Geometry: final body of the model. Coordinates: model frame, mm. Give positions to 0.01 mm unless a question says otherwise; leave off trailing zeros. Order: outer loops, then holes, each group sorted by start corner. A loop starts at its lowest first (then second) coordinate and runs counter-clockwise, first axis right, second up. Notation, with made-up numbers: M 75.25,74.25 L 106.25,74.25 A26 cw 106.25,96.25 Z; hole C 88,-24.5 d11. An arc over 180 degrees is marked long. Use CSV: the item, a comma, the result in double quotes.
Autodesk Inventor part; units mm, degrees
ref_plane "YZ Plane" through (0, 0, 0) normal (1, 0, 0) x (0, 1, 0)
ref_plane "XZ Plane" through (0, 0, 0) normal (0, 1, 0) x (-1, 0, 0)
ref_plane "XY Plane" through (0, 0, 0) normal (0, 0, 1) x (1, 0, 0)
sketch "スケッチ1" plane through (0, 0, 0) normal (0, 1, 0) x (-1, 0, 0)
  line L0 (127.92, 0) -> (-21.32, 0)
  line L1 (0, -84) -> (0, 84)
  line L2 (106.6, 0) -> (106.6, -60)
  line L3 (106.6, -60) -> (0, -60)
  line L4 (0, -40) -> (86.6, -40)
  line L5 (86.6, -40) -> (86.6, 0)
  line L6 (106.6, 0) -> (106.6, 60)
  line L7 (106.6, 60) -> (0, 60)
  line L8 (0, 40) -> (86.6, 40)
  line L9 (86.6, 40) -> (86.6, 0)
  line L10 (0, 60) -> (0, 40)
  line L11 (0, -40) -> (0, -60)
  point P0 (0, 0)
  dimension "d0" = 20
  dimension "d4" = 20
  dimension "d15" = 60
  dimension "d16" = 106.6
extrude "押し出し1" add sketch "スケッチ1" along normal blind 5 contours L2 L3 L1 L4 L5 L0 | L0 L9 L8 L1 L7 L6
sketch "スケッチ2" plane through (0, 5, 0) normal (0, 1, 0) x (1, 0, 0)
  circle A0 centre (-10, -50) radius 5
  line L0 (0, -60) -> (0, -40)
  line L1 (-106.6, -60) -> (0, -60)
  line L2 (-127.92, 0) -> (21.32, 0)
  circle A1 centre (-10, 50) radius 5
  circle A2 centre (-96.6, 0) radius 5
  line L3 (-86.6, -40) -> (-86.6, 40)
  point P0 (0, 0)
  dimension "d8" = 10
  dimension "d9" = 10
  dimension "d10" = 10
  dimension "d11" = 10
  dimension "d12" = 10
extrude "押し出し2" cut sketch "スケッチ2" against normal blind 5
properties part number "bogie_square" material "アルミニウム 6061"
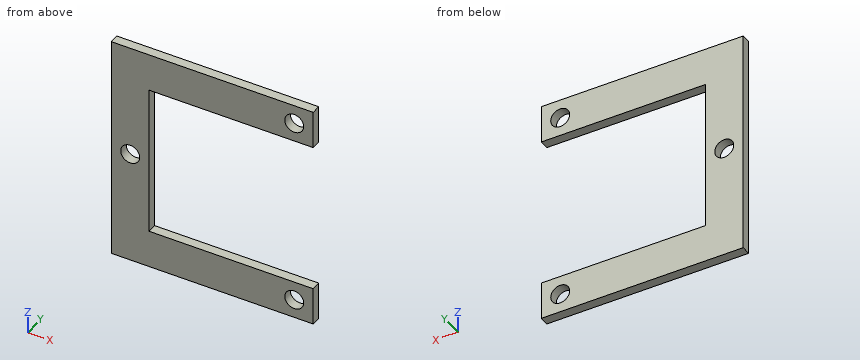
1. Line query: line 1 (Z direction, x = -10, y = 1.75); line 2 (Z direction, x = -96.6, y = 1.5); line 3 (Z direction, x = -52, y = 3.5). Output: solid intervals per line, ascending.
Answer:
line 1,"-60 to -55, -45 to -40, 40 to 45, 55 to 60"
line 2,"-60 to -5, 5 to 60"
line 3,"-60 to -40, 40 to 60"
2. Pin query (flat end, axial travel): pin 1 Ø1 at (y, z) = (2, -5.5) entering from +X; pin 2 Ø9 at (x, z) = (-10, 50) entering from -Y. Return the tip coordinate at first contact, or that it passes through.
Answer:
pin 1,"x = -86.6"
pin 2,"through"
3. Section B-B, the plane x = -10. Return the cut outline in (y, z).
Answer:
outline,"M 0,-60 L 5,-60 L 5,-55 L 0,-55 Z; M 0,-45 L 5,-45 L 5,-40 L 0,-40 Z; M 0,40 L 5,40 L 5,45 L 0,45 Z; M 0,55 L 5,55 L 5,60 L 0,60 Z"
4. Section D-D, the plane x = -96.6. Return the cut outline in (y, z).
Answer:
outline,"M 0,-60 L 5,-60 L 5,-5 L 0,-5 Z; M 0,5 L 5,5 L 5,60 L 0,60 Z"
5. Section A-A, the plane z = 50. Return the cut outline in (x, y).
Answer:
outline,"M -106.6,0 L -15,0 L -15,5 L -106.6,5 Z; M -5,0 L 0,0 L 0,5 L -5,5 Z"
6. Section C-C, the plane y = 1.75. Return the cut outline in (x, z).
Answer:
outline,"M -106.6,-60 L 0,-60 L 0,-40 L -86.6,-40 L -86.6,40 L 0,40 L 0,60 L -106.6,60 Z; hole C -96.6,0 d10; hole C -10,-50 d10; hole C -10,50 d10"
